Design review of the part built by this model. Coordinates are the model's own, in mm. Face numbers are marked on the shaded views. A direction names the side the tool comes from. Coordinates: 2 decimals unless noted, no trailing zeros. Loops run counter-clockwise (first coordinate to the right, second up) from the corner with the lowest first, then second, coordinate; pieces in that order, holes last. Notation, with made-up numbers: (37, -5.75) - (86, -5.75) arc R23 cw to (86, 31.25) - close; hole circle Ø5 at (65.5, -37.75). An arc over 180 degrees is marked (long way). Answer in a Markdown table with one row per item. Add a question column.
(1) Clearance check with flat-ended pins moving along their axes: pin 1 (3 mm diameter, centred on x = -1.5, y = 12, fed in from -Z); pin 2 (4 mm diameter, centred on x = -0.5, z = -0.5, fed in from -Y); pin 3 (2.5 mm diameter, centred on x = 0, z = 0, fed in from -Y); pin 4 (1 mm diameter, centred on x = -1.5, y = 3, fed in from +Z). State where each tip first meets the part, or that it passes through.
(2) For the marked faces 4, 5 and 6, list the 3-axis set-ups (+Z, -Z, +X, -X, +Y, -Y) from which the entire face can be reached by the end or side of a thin tool; tool diameter is ignored.
(3) We need section B-B, the plane x = 0.25. Write out the cut boundary in (y, z), plus the area to 3 significant figures.
(4) We need section C-C, the plane z = -2.75. Write out the cut boundary in (x, y), plus the area to 3 significant figures.
(5) The part is to be moulded in two halves that separate along Z. For the marked faces 1, 2 and 3, say which applies: released by +Z, released by -Z, zero draft, split by the parting line, or undercut.
(6) We need section D-D, the plane y = 3.75. Write out the cut boundary in (x, z).
(7) To check wall thickness, follow L1, parallel to Z at x = 0, y = 11; L2, parallel to X at y = 13.5, z = 1.25. State the ranges of each line that lie inside material, in increasing order. Write a range as [from, to].
(8) We need section A-A, the plane y = 2. Write out the cut boundary in (x, z), plus the area to 3 significant figures.
Autodesk Inventor part; units mm, degrees
ref_plane "YZ Plane" through (0, 0, 0) normal (1, 0, 0) x (0, 1, 0)
ref_plane "XZ Plane" through (0, 0, 0) normal (0, 1, 0) x (-1, 0, 0)
ref_plane "XY Plane" through (0, 0, 0) normal (0, 0, 1) x (1, 0, 0)
sketch "Náčrt1" plane through (0, 0, 0) normal (0, 1, 0) x (-1, 0, 0)
  circle A0 centre (0, 0) radius 4
  dimension "nutOuterDia" = 8
extrude "Vysunutí2" add sketch "Náčrt1" along normal blind 16
sketch "Náčrt3" plane through (0, 0, 0) normal (0, -1, 0) x (1, 0, 0)
  circle A0 centre (0, 0) radius 4
  line L0 (-2.8868, 0) -> (-1.4434, 2.5)
  line L1 (-1.4434, 2.5) -> (1.4434, 2.5)
  line L2 (1.4434, 2.5) -> (2.8868, 0)
  line L3 (2.8868, 0) -> (1.4434, -2.5)
  line L4 (1.4434, -2.5) -> (-1.4434, -2.5)
  line L5 (-1.4434, -2.5) -> (-2.8868, 0)
  dimension "keyHoleSize" = 5
extrude "Vysunutí3" cut sketch "Náčrt3" against normal blind 3 contours L0 L1 L2 L3 L4 L5
sketch "Náčrt4" plane through (0, 16, 0) normal (0, 1, 0) x (1, 0, 0)
  circle A0 centre (0, 0) radius 4
  circle A1 centre (0, 0) radius 3
extrude "Vysunutí4" cut sketch "Náčrt4" against normal blind 13
sketch "Náčrt5" plane through (0, 16, 0) normal (0, 1, 0) x (1, 0, 0)
  circle A0 centre (0, 0) radius 3
  circle A1 centre (0, 0) radius 2
extrude "Vysunutí5" cut sketch "Náčrt5" against normal blind 10 contours A1
thread "Závit2"
properties part number "nut"
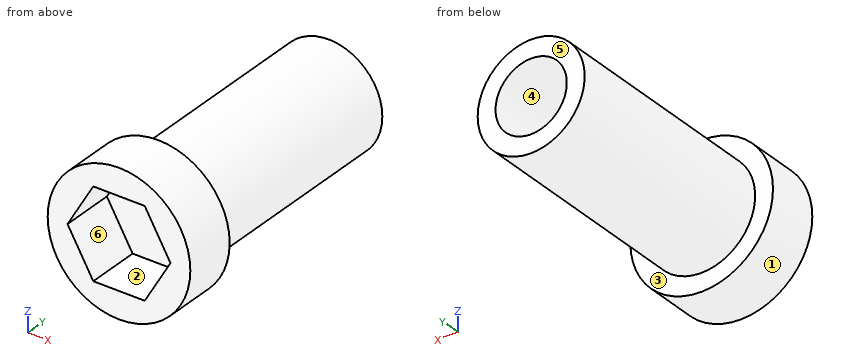
Responses:
| question | item | result |
|---|---|---|
| 1 | pin 1 | stops at z = -3 |
| 1 | pin 2 | stops at y = 0 |
| 1 | pin 3 | stops at y = 3 |
| 1 | pin 4 | stops at z = 3.87 |
| 2 | face 4 | +Y |
| 2 | face 5 | +Z, -Z, +X, -X, +Y |
| 2 | face 6 | -Y |
| 3 | outline | (0, -3.99) - (3, -3.99) - (3, -2.99) - (16, -2.99) - (16, -1.98) - (6, -1.98) - (6, 1.98) - (16, 1.98) - (16, 2.99) - (3, 2.99) - (3, 3.99) - (0, 3.99) - (0, 2.5) - (3, 2.5) - (3, -2.5) - (0, -2.5) - close |
| 3 | area | 47.0 mm2 |
| 4 | outline | (-2.9, 0) - (2.9, 0) - (2.9, 3) - (1.2, 3) - (1.2, 16) - (-1.2, 16) - (-1.2, 3) - (-2.9, 3) - close |
| 4 | area | 48.6 mm2 |
| 5 | face 1 | split by the parting line |
| 5 | face 2 | undercut |
| 5 | face 3 | zero draft |
| 6 | outline | circle Ø6 at (0, 0) |
| 7 | L1 | z = [-3, -2], [2, 3] |
| 7 | L2 | x = [-2.73, -1.56], [1.56, 2.73] |
| 8 | outline | circle Ø8 at (0, 0); hole (-2.89, 0) - (-1.44, -2.5) - (1.44, -2.5) - (2.89, 0) - (1.44, 2.5) - (-1.44, 2.5) - close |
| 8 | area | 28.6 mm2 |
